Print and shaded views of the part. All mm, measured from the part's lowest x, y and z. A direction names the side the tool comes from. Coordinates: 2 decimals unless noted, no trailing zeros. Loops run counter-clockwise (first coordinate to the right, second up) from the corner with the lowest first, then second, coordinate; pieces in that order, holes last. Notation, with made-up numbers: M -8.5,-39 L 31.5,-39 A16 ccw 31.5,-15 Z; hole C -19,-14.75 d1. An arc over 180 degrees is marked long. Answer as CSV lines item,"result". Start each with the question number.
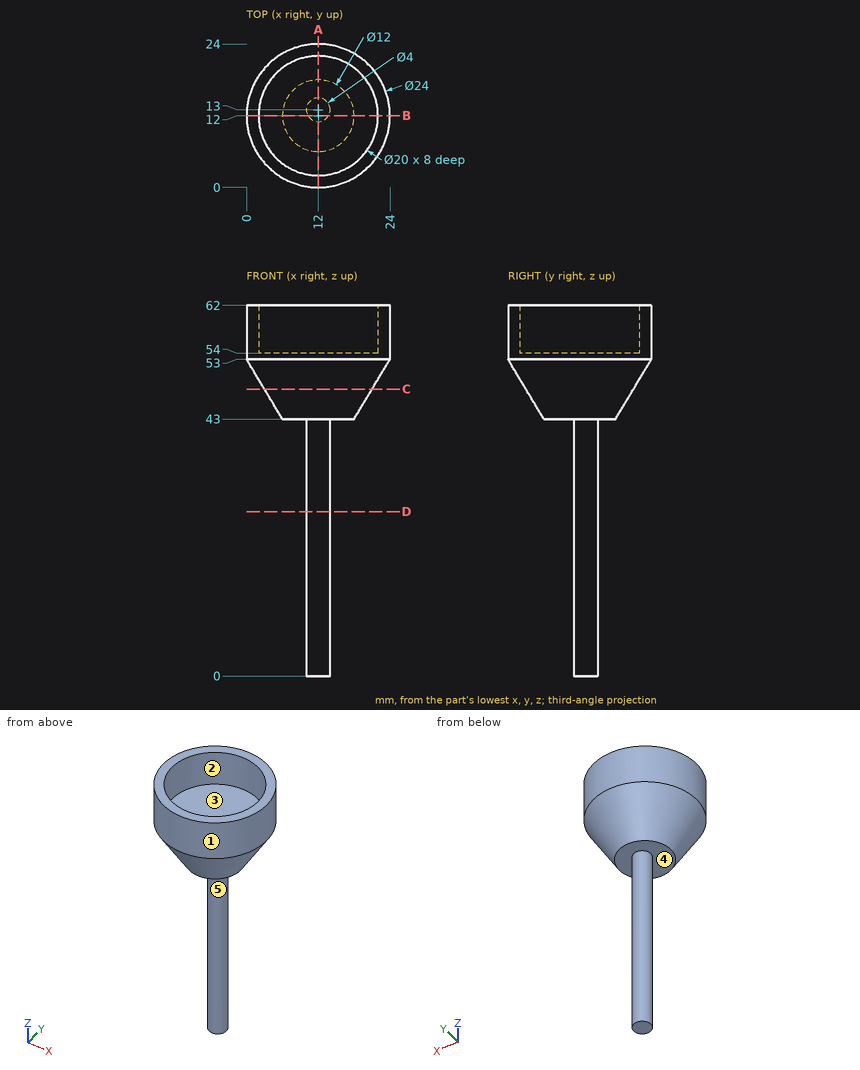
Q1. Tool access for the marked faces 1 and 2: list every direction of +Z, -Z, +X, -X, +Y, -Y with a clear straight run to the whole face (end or side of a thin tool).
Q2. Slice it at D-D, the plane z = 27.5. Write the cut outline in (x, y), and give its area (3 significant figures).
Q3. Slice it at C-C, the plane z = 48. Write the cut outline in (x, y), and give its area (3 significant figures).
Q4. Flat gauge pins, fed straight in: P1, Ø10, axis at y = 19.5, z = 9.5, coming from the +X side; P2, Ø1.5, axis at y = 10.5, z = 40.5, coming from the -X side; P3, Ø6, axis at y = 13.5, z = 27.5, coming from the -X side. Where does each tip first touch, or does it go through?
Q5. Two-plate mould, pull along Y, no slides. Class the marked faces 3, 4 and 5: +Y half, -Y half, draft (parallel to the pull), parting line (faces both ways), or undercut.
Q6. Slice it at A-A, the plane x = 12. Write the cut outline in (y, z).
Q7. Slice it at B-B, the plane y = 12. Write the cut outline in (x, z), and give its area (3 significant figures).
Q8. Wall check: L1, parallel to Y at x = 12, z = 58.5; L2, parallel to Z at x = 7.75, y = 10.75; L3, parallel to X at y = 2.5, z = 52. Give the ranges that are in metal, low to high.
Solved:
1,face 1,"+Z, -Z"
1,face 2,"+Z"
2,outline,"C 12,13 d4"
2,area,"12.6 mm2"
3,outline,"C 12,12 d18"
3,area,"254 mm2"
4,P1,"stops at x = 13.32"
4,P2,"stops at x = 11.03"
4,P3,"stops at x = 10"
5,face 3,"undercut"
5,face 4,"draft"
5,face 5,"parting line"
6,outline,"M 0,53 L 6,43 L 11,43 L 11,0 L 15,0 L 15,43 L 18,43 L 24,53 L 24,62 L 22,62 L 22,54 L 2,54 L 2,62 L 0,62 Z"
7,outline,"M 0,53 L 6,43 L 10.27,43 L 10.27,0 L 13.73,0 L 13.73,43 L 18,43 L 24,53 L 24,62 L 22,62 L 22,54 L 2,54 L 2,62 L 0,62 Z"
7,area,"385 mm2"
8,L1,"y = 0 to 2, 22 to 24"
8,L2,"z = 43 to 54"
8,L3,"x = 5.7 to 18.3"
